Autodesk Inventor part; units mm, degrees
ref_plane "YZ Plane" through (0, 0, 0) normal (1, 0, 0) x (0, 1, 0)
ref_plane "XZ Plane" through (0, 0, 0) normal (0, 1, 0) x (-1, 0, 0)
ref_plane "XY Plane" through (0, 0, 0) normal (0, 0, 1) x (1, 0, 0)
sketch "Sketch1" plane through (0, 0, 0) normal (0, 0, 1) x (1, 0, 0)
  circle A0 centre (0, 0) radius 6.35
  circle A1 centre (0, 25.4) radius 4.7625
  line L0 (0, 25.4) -> (0, 0)
  line L1 (-4.7532, 25.6977) -> (-6.3376, 0.3969)
  line L2 (6.3376, 0.3969) -> (4.7532, 25.6977)
  dimension "d0" = 12.7
  dimension "d1" = 9.525
  dimension "d2" = 25.4
extrude "Extrusion1" add sketch "Sketch1" along normal blind 6.35
sketch "Sketch2" plane through (0, 0, 6.35) normal (0, 0, 1) x (1, 0, 0)
  arc A0 (-6.3376, 0.3969) -> (6.3376, 0.3969) centre (0, 0) ccw
  circle A1 centre (0, 0) radius 3.175
  dimension "d5" = 6.35
extrude "Extrusion2" cut sketch "Sketch2" against normal through all
sketch "Sketch3" plane through (0, 0, 6.35) normal (0, 0, 1) x (1, 0, 0)
  arc A0 (4.7532, 25.6977) -> (-4.7532, 25.6977) centre (0, 25.4) ccw
  circle A1 centre (0, 25.4) radius 3.175
  dimension "d8" = 6.35
extrude "Extrusion3" add sketch "Sketch3" along normal blind 19.05
properties part number "Crank Handle" material "PPS Plastic"
Geometry: final body of the model. Coordinates: model frame, mm. A direction names the side the tool comes from. Coordinates: 2 decimals unless noted, no trailing zeros. Order: outer loops, then holes, each group sorted by start corner. A loop starts at its lowest first (then second) coordinate and runs counter-clockwise, first axis right, second up. Notation, with made-up numbers: (-32, 64) - (23, 64) arc R14 cw to (23, 81) - close; hole circle Ø10 at (62.5, 8). An arc over 180 degrees is marked (long way). Use one line per item in the form item = value.
1) Pin query (flat end, axial travel): pin 1 (5 mm diameter, centred on y = 15.5, z = 10, fed in from -X); pin 2 (1.5 mm diameter, centred on x = -3, z = 18, fed in from +Y); pin 3 (8 mm diameter, centred on y = 11, z = 6, fed in from +X); pin 4 (4 mm diameter, centred on x = -1, z = 9, fed in from +Y) (3 decimals). Return the tip coordinate at first contact, or that it passes through.
Solutions:
pin_1 = through
pin_2 = 27.64
pin_3 = 5.92
pin_4 = 28.575
2) Section A-A (y = 0). Return loops of the section in (x, z) (3 decimals).
Solutions:
outline = (-6.35, 0) - (-3.175, 0) - (-3.175, 6.35) - (-6.35, 6.35) - close; (3.175, 0) - (6.35, 0) - (6.35, 6.35) - (3.175, 6.35) - close
3) Ray query, L1, parallel to Z at x = 3.75, y = 3; L2, parallel to Y at x = -0.5, z = 5.5; L3, parallel to Y at x = 1.75, z = 12.25. Return the intervals inside material, ascending.
Solutions:
L1 = 0 to 6.35
L2 = -6.33 to -3.14, 3.14 to 30.14
L3 = 22.75 to 28.05
4) Section D-D (z = 20). Return loops of the section in (x, y) (3 decimals), then the cut area to 3 significant figures.
Solutions:
outline = circle Ø6.35 at (0, 25.4)
area = 31.7 mm^2
5) Section B-B (x = 0.75). Return loops of the section in (y, z).
Solutions:
outline = (-6.31, 0) - (-3.09, 0) - (-3.09, 6.35) - (-6.31, 6.35) - close; (3.09, 0) - (30.1, 0) - (30.1, 6.35) - (28.49, 6.35) - (28.49, 25.4) - (22.31, 25.4) - (22.31, 6.35) - (3.09, 6.35) - close
6) Set-up query: faces 4 (the face through (-5.534, 13.224, 3.131)), 5 (the face through (-0.41, 22.25, 15.74)). Return all of +Z, -Z, +X, -X, +Y, -Y with unobstructed straight access to the full face (end or side cutting, diameter ignored); none if empty.
Solutions:
face_4 = +Z, -Z, -X, +Y
face_5 = +Z
7) Mould query, pull axis X, two halves, no side actions, for faces 1 (the face through (-0.1, 30.16, 3.13)), 2 (the face through (5.556, 12.87, 3.131)), 3 (the face through (-0.69, -3.1, 3.22)). Classes: +X half, -X half, draft (parallel to the pull), parting line (faces both ways), or undercut.
Solutions:
face_1 = parting line
face_2 = +X half
face_3 = undercut
